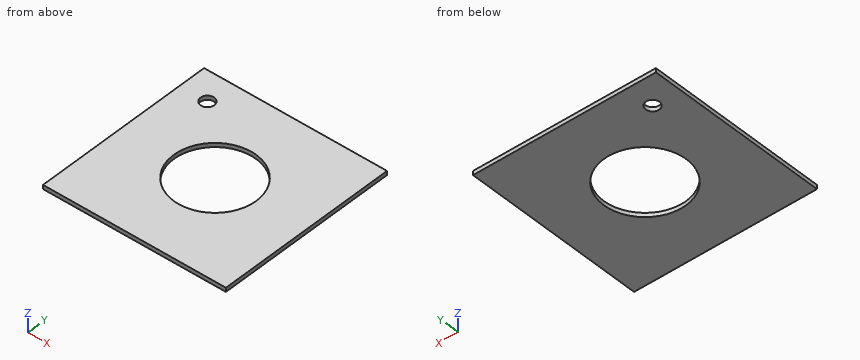
from build123d import *

# Parameters (mm, degrees)
F0_W     = 222.25
F0_H     = 222.25
F1_DEPTH = 5
F2_R     = 50
F3_DEPTH = 5.001
F4_R     = 8.334375
F5_DEPTH = 5.001


with BuildPart() as f1:
    # F0 (on Top) → F1 (new body)
    with BuildSketch(Plane.XY):
        Rectangle(F0_W, F0_H)
    extrude(amount=F1_DEPTH)

    # F2 (on face) → F3 (cut, through all)
    with BuildSketch(Plane.XY.offset(5)):
        Circle(F2_R)
    extrude(amount=-F3_DEPTH, mode=Mode.SUBTRACT)

    # F4 (on face) → F5 (cut, through all)
    with BuildSketch(Plane.XY.offset(5)):
        with Locations((-77.390625, 77.390625)):
            Circle(F4_R)
    extrude(amount=-F5_DEPTH, mode=Mode.SUBTRACT)


solid = f1.part
For this review, take the finished solid that the model builds, in its own axes (mm). Coordinates: 2 decimals unless noted, no trailing zeros. Order: outer loops, then holes, each group sorted by start corner. A loop starts at its lowest first (then second) coordinate and runs counter-clockwise, first axis right, second up. Notation, with made-up numbers: (11, 82.5) -> (62, 82.5) arc R20 cw to (62, 120.5) -> close; hole circle Ø9 at (-29.75, 32.25). An arc over 180 degrees is marked (long way). Return JSON: item names as keys, results as strings.
1. We need section C-C on z = 3.55. Write out the cut boundary in (x, y) (3 decimals).
Answer block:
{"outline": "(-111.125, -111.125) -> (111.125, -111.125) -> (111.125, 111.125) -> (-111.125, 111.125) -> close; hole circle Ø16.669 at (-77.391, 77.391); hole circle Ø100 at (0, 0)"}
2. We need section A-A on y = 0. Write out the cut boundary in (x, z) (3 decimals).
Answer block:
{"outline": "(-111.125, 0) -> (-50, 0) -> (-50, 5) -> (-111.125, 5) -> close; (50, 0) -> (111.125, 0) -> (111.125, 5) -> (50, 5) -> close"}
3. For line 1 (Y direction, x = 0, z = 3.8) (3 decimals); line 2 (X direction, y = 10.5, z = 4.35) (3 decimals); line 3 (X direction, y = -29, z = 2.2) (3 decimals), list the stretches that pass through material, from the lowest coordinate up. Write a range as from..to.
Answer block:
{"line 1": "-111.125..-50, 50..111.125", "line 2": "-111.125..-48.885, 48.885..111.125", "line 3": "-111.125..-40.731, 40.731..111.125"}
